Source: CAD feature listing. Evaluate the final solid. Frame: model axes, mm. A direction names the side the tool comes from. Round coordinates to 2 decimals unless told otherwise and drop trailing zeros. Order: outer loops, then holes, each group sorted by start corner. A loop starts at its lowest first (then second) coordinate and runs counter-clockwise, first axis right, second up. Notation, with made-up numbers: M 80.5,-17 L 118.5,-17 A24 ccw 118.5,20 Z; hole C 36,-8.75 d7. An arc over 180 degrees is marked long. Use one line per item in the form item = value. Start each with the question number.
Q1. Material intervals for probe 1 along X at (y, z) = (1.3, -44); probe 2 along Z at (x, y) = (-10.5, 0.3); probe 3 along Z at (x, y) = (-29, 0.1), sorted ascending.
Q2. Reachability of faces 1 (the flat face through (-11, 0.78, 3.49)), 2 (the cylindrical face through (-40.2, 0.8, 16.5)) from +Z, -Z, +X, -X, +Y, -Y: full face, straight path, thin tool, end or side. Return the list, or none.
Q3. Section A-A (x = 0). Return the cut outline in (y, z).
Q4. Pull-direction query (X, two-part tool) for faces 3 (the flat face through (-10.7, 0.8, -32.1)), 4 (the flat face through (-13, 1.588, 9)), 5 (the cylindrical face through (-36.088, 0.783, -43.358)); classes: pulls with the +X half, pulls with the -X half, needs draft (parallel to the pull), parting line crosses it, or undercut.
Q5. Contact query for a flat-ended pin moving along its axis: pin 1 (2.5 mm diameter, centred on x = -11.4, z = 38.99, fed in from +Y). Output: stop coordinate, or through.
Q6. Section D-D (z = -34.5). Return the cut outline in (x, y).
Q7. Section B-B (x = -33.5). Return the cut outline in (y, z), plus the area to 3 significant figures.
Q8. Section C-C (y = 0.3). Give the number of separate pieces and of enclosed holes in the cut face, plus the area to 3 significant figures.
Autodesk Inventor part; units mm, degrees
ref_plane "YZ Plane" through (0, 0, 0) normal (1, 0, 0) x (0, 1, 0)
ref_plane "XZ Plane" through (0, 0, 0) normal (0, 1, 0) x (-1, 0, 0)
ref_plane "XY Plane" through (0, 0, 0) normal (0, 0, 1) x (1, 0, 0)
sketch "main_gusset" plane through (0, 0, 0) normal (0, 0, 1) x (1, 0, 0)
  circle A0 centre (-10.4381, -28.24) radius 2.1844
  arc A1 (-15.3966, -32.2068) -> (-10.4381, -34.59) centre (-10.4381, -28.24) ccw
  circle A2 centre (-23.1381, -12.365) radius 2.0955
  line L0 (-16.7881, 12.8688) -> (-16.7881, -9.0238)
  line L1 (-29.4881, 16.21) -> (-29.4881, -12.365)
  arc A3 (-16.7881, -9.0238) -> (-16.0924, -11.0072) centre (-13.6131, -9.0238) ccw
  arc A4 (-29.4881, -12.365) -> (-28.0966, -16.3318) centre (-23.1381, -12.365) ccw
  line L2 (-16.0924, -11.0072) -> (-8.3394, -20.6984)
  arc A5 (-8.3394, -20.6984) -> (-5.8602, -21.89) centre (-5.8602, -18.715) ccw
  line L3 (-28.0966, -16.3318) -> (-15.3966, -32.2068)
  line L4 (-10.4381, -34.59) -> (14.9619, -34.59)
  circle A6 centre (-10.4381, 32.085) radius 2.1844
  circle A7 centre (14.9619, 32.0717) radius 2.1844
  arc A8 (-10.4381, 38.435) -> (-15.3966, 36.0518) centre (-10.4381, 32.085) ccw
  arc A9 (14.3804, 25.735) -> (14.9619, 38.435) centre (14.9619, 32.0717) ccw
  line L5 (14.9619, 38.435) -> (-10.4381, 38.435)
  circle A10 centre (-23.1381, 16.21) radius 2.0955
  line L6 (14.9619, 25.735) -> (-5.8602, 25.735)
  arc A11 (-16.0924, 14.8522) -> (-16.7881, 12.8688) centre (-13.6131, 12.8688) ccw
  arc A12 (-28.0966, 20.1768) -> (-29.4881, 16.21) centre (-23.1381, 16.21) ccw
  line L7 (-8.3394, 24.5434) -> (-16.0924, 14.8522)
  arc A13 (-5.8602, 25.735) -> (-8.3394, 24.5434) centre (-5.8602, 22.56) ccw
  line L8 (-28.0966, 20.1768) -> (-15.3966, 36.0518)
  circle A14 centre (14.9619, -28.24) radius 2.1844
  arc A15 (14.9619, -34.59) -> (14.9619, -21.89) centre (14.9619, -28.24) ccw
  line L9 (-5.8602, -21.89) -> (14.9619, -21.89)
  line L10 (0.0267, 34.3202) -> (4.4971, 34.3202)
  line L11 (4.4971, 34.3202) -> (4.4971, 29.8498)
  line L12 (4.4971, 29.8498) -> (0.0267, 29.8498)
  line L13 (0.0267, 29.8498) -> (0.0267, 34.3202)
  line L14 (0.0267, 34.3202) -> (4.4971, 29.8498) construction
  line L15 (4.4971, 34.3202) -> (0.0267, 29.8498) construction
  line L16 (0.0267, -26.0048) -> (4.4971, -26.0048)
  line L17 (4.4971, -26.0048) -> (4.4971, -30.4752)
  line L18 (4.4971, -30.4752) -> (0.0267, -30.4752)
  line L19 (0.0267, -30.4752) -> (0.0267, -26.0048)
  line L20 (0.0267, -26.0048) -> (4.4971, -30.4752) construction
  line L21 (4.4971, -26.0048) -> (0.0267, -30.4752) construction
  point P0 (-1.5323, 2.5213)
  point P1 (2.2619, 32.085)
  point P2 (2.2619, -28.24)
  dimension "d0" = 12.7
  dimension "d1" = 12.7
  dimension "d2" = 12.7
  dimension "d3" = 3.175
  dimension "d6" = 4.4704
  dimension "d7" = 4.4704
  dimension "d8" = 4.4704
  dimension "d9" = 4.4704
  dimension "d10" = 12.7
  dimension "d11" = 12.7
  dimension "d12" = 6.35
  dimension "d13" = 6.35
  dimension "d14" = 15.875
  dimension "d15" = 15.875
  dimension "d16" = 12.7
sketch "Sketch1" plane through (0, 0, 0) normal (0, 1, 0) x (-1, 0, 0)
  arc A0 (15.5751, 43.7797) -> (5.2982, 40.7397) centre (11.4031, 38.9925) ccw
  line L0 (42.3791, 20.4205) -> (15.5751, 43.7797)
  line L1 (-6.3499, 0.0397) -> (5.2982, 40.7397)
  circle A1 centre (11.4031, 38.9925) radius 2.1844
  arc A2 (15.5751, 43.7797) -> (5.2982, 40.7397) centre (11.4031, 38.9925) ccw
  circle A3 centre (12.422, -44.5285) radius 2.1844
  arc A4 (7.4388, -48.4642) -> (12.3823, -50.8784) centre (12.422, -44.5285) ccw
  circle A5 centre (-0.1786, -28.5744) radius 2.0955
  line L2 (6.329, -3.3808) -> (6.1922, -25.273)
  line L3 (-6.3499, 0.0397) -> (-6.5284, -28.5348)
  arc A6 (6.1922, -25.273) -> (6.8755, -27.2607) centre (9.3671, -25.2928) ccw
  arc A7 (-6.5284, -28.5348) -> (-5.1618, -32.5102) centre (-0.1786, -28.5744) ccw
  line L4 (6.8755, -27.2607) -> (14.5678, -37.0002)
  arc A8 (14.5678, -37.0002) -> (17.0395, -38.2072) centre (17.0594, -35.0323) ccw
  line L5 (-5.1618, -32.5102) -> (7.4388, -48.4642)
  line L6 (12.3823, -50.8784) -> (37.7818, -51.0371)
  circle A9 centre (12.799, 15.7953) radius 2.1844
  circle A10 centre (38.1984, 15.6233) radius 2.1844
  arc A11 (12.8386, 22.1452) -> (7.8653, 19.793) centre (12.799, 15.7953) ccw
  arc A12 (37.5773, 9.2904) -> (38.2381, 21.9865) centre (38.1984, 15.6233) ccw
  line L7 (38.2381, 21.9865) -> (12.8386, 22.1452)
  circle A13 centre (0, 0) radius 2.0955
  line L8 (38.1588, 9.2867) -> (17.3371, 9.4168)
  arc A14 (7.0371, -1.4018) -> (6.329, -3.3808) centre (9.5039, -3.4006) ccw
  arc A15 (-4.9336, 3.9977) -> (-6.3499, 0.0397) centre (0, 0) ccw
  line L9 (14.8505, 8.2408) -> (7.0371, -1.4018)
  arc A16 (17.3371, 9.4168) -> (14.8505, 8.2408) centre (17.3173, 6.2419) ccw
  line L10 (-4.9336, 3.9977) -> (7.8653, 19.793)
  circle A17 centre (37.8215, -44.6872) radius 2.1844
  arc A18 (37.7818, -51.0371) -> (37.8612, -38.3374) centre (37.8215, -44.6872) ccw
  line L11 (17.0395, -38.2072) -> (37.8612, -38.3374)
  line L12 (23.2775, 17.9651) -> (27.7478, 17.9371)
  line L13 (27.7478, 17.9371) -> (27.7199, 13.4668)
  line L14 (27.7199, 13.4668) -> (23.2496, 13.4948)
  line L15 (23.2496, 13.4948) -> (23.2775, 17.9651)
  line L16 (23.2775, 17.9651) -> (27.7199, 13.4668) construction
  line L17 (27.7478, 17.9371) -> (23.2496, 13.4948) construction
  line L18 (22.9005, -42.3587) -> (27.3708, -42.3867)
  line L19 (27.3708, -42.3867) -> (27.3429, -46.857)
  line L20 (27.3429, -46.857) -> (22.8726, -46.8291)
  line L21 (22.8726, -46.8291) -> (22.9005, -42.3587)
  line L22 (22.9005, -42.3587) -> (27.3429, -46.857) construction
  line L23 (27.3708, -42.3867) -> (22.8726, -46.8291) construction
  point P0 (0, 0)
  point P1 (42.3791, 20.4205)
  point P2 (-6.3499, 0.0397)
  point P3 (-5.4094, 3.3258)
  point P4 (-6.3499, 0.0397)
  dimension "d18" = 12.7
extrude "Extrusion1" add sketch "Sketch1" along normal blind 1.5875
properties part number "funnel_gusset" material "Acetal Resin, White"
Results list:
q1.probe_1 = -44.13 to -39.89, -35.75 to -27.36, -22.89 to -14.54, -10.3 to -3.91
q1.probe_2 = -50.58 to -45.57, -43.49 to -31.85, 2.87 to 37, 40.98 to 45.28
q1.probe_3 = -50.98 to -38.28, 9.34 to 32.08
q2.face_1 = -X, +Y, -Y
q2.face_2 = +Y, -Y
q3.outline = M 0,-39.05 L 1.59,-39.05 L 1.59,-30.66 L 0,-30.66 Z; M 0,-26.49 L 1.59,-26.49 L 1.59,-2.1 L 0,-2.1 Z; M 0,2.1 L 1.59,2.1 L 1.59,22.23 L 0,22.23 Z
q4.face_3 = pulls with the -X half
q4.face_4 = needs draft
q4.face_5 = undercut
q5.pin_1 = through
q6.outline = M -12.59,0 L 3.59,0 L 3.59,1.59 L -12.59,1.59 Z
q7.outline = M 0,-51.01 L 1.59,-51.01 L 1.59,-38.31 L 0,-38.31 Z; M 0,9.32 L 1.59,9.32 L 1.59,28.16 L 0,28.16 Z
q7.area = 50.1 mm2
q8.separate_pieces = 1
q8.enclosed_holes = 9
q8.area = 2,150 mm2
